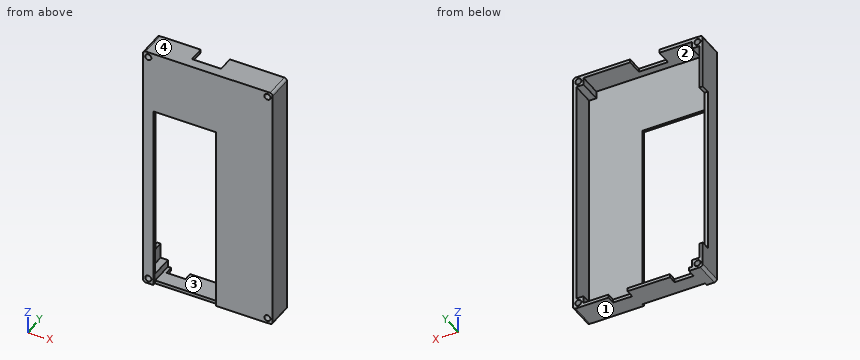
Autodesk Inventor part; units mm, degrees
ref_plane "YZ Plane" through (0, 0, 0) normal (1, 0, 0) x (0, 1, 0)
ref_plane "XZ Plane" through (0, 0, 0) normal (0, 1, 0) x (-1, 0, 0)
ref_plane "XY Plane" through (0, 0, 0) normal (0, 0, 1) x (1, 0, 0)
sketch "Sketch1" plane through (0, 0, 0) normal (0, 1, 0) x (-1, 0, 0)
  line L0 (0, 0) -> (62.23, 0)
  line L1 (62.23, 0) -> (62.23, -120.65)
  line L2 (62.23, -120.65) -> (0, -120.65)
  line L3 (0, -120.65) -> (0, 0)
  dimension "d0" = 62.23
  dimension "d1" = 120.65
extrude "Extrusion1" add sketch "Sketch1" along normal blind 1.5
sketch "Sketch2" plane through (0, 1.5, 0) normal (0, 1, 0) x (1, 0, 0)
  line L0 (-60.6425, 1.5875) -> (-1.5875, 1.5875)
  line L1 (-1.5875, 1.5875) -> (-1.5875, 119.0625)
  line L2 (-1.5875, 119.0625) -> (-60.6425, 119.0625)
  line L3 (-60.6425, 119.0625) -> (-60.6425, 1.5875)
  line L4 (-62.23, 0) -> (0, 0)
  line L5 (0, 0) -> (0, 120.65)
  line L6 (-62.23, 120.65) -> (-62.23, 0)
  line L7 (0, 120.65) -> (-62.23, 120.65)
  line L8 (0, 0) -> (-5.08, 0)
  line L9 (-5.08, 0) -> (-5.08, 5.08)
  line L10 (-5.08, 5.08) -> (0, 5.08)
  line L11 (0, 5.08) -> (0, 0)
  line L12 (-62.23, 0) -> (-57.15, 0)
  line L13 (-57.15, 0) -> (-57.15, 5.08)
  line L14 (-57.15, 5.08) -> (-62.23, 5.08)
  line L15 (-62.23, 5.08) -> (-62.23, 0)
  line L16 (0, 120.65) -> (-5.08, 120.65)
  line L17 (-5.08, 120.65) -> (-5.08, 115.57)
  line L18 (-5.08, 115.57) -> (0, 115.57)
  line L19 (0, 115.57) -> (0, 120.65)
  line L20 (-62.23, 120.65) -> (-57.15, 120.65)
  line L21 (-57.15, 120.65) -> (-57.15, 115.57)
  line L22 (-57.15, 115.57) -> (-62.23, 115.57)
  line L23 (-62.23, 115.57) -> (-62.23, 120.65)
  point P0 (0, 115.57)
  point P1 (-1.5875, 115.57)
  point P2 (-1.5875, 5.08)
  point P3 (-5.08, 1.5875)
  point P4 (-57.15, 1.5875)
  point P5 (-60.6425, 5.08)
  point P6 (-5.08, 119.0625)
  point P7 (-60.6425, 115.57)
  point P8 (-57.15, 119.0625)
  dimension "d4" = 1.5875
  dimension "d5" = 1.5875
  dimension "d6" = 1.5875
  dimension "d7" = 1.5875
  dimension "d8" = 5.08
  dimension "d9" = 5.08
  dimension "d10" = 5.08
  dimension "d11" = 5.08
  dimension "d12" = 5.08
  dimension "d13" = 5.08
  dimension "d14" = 5.08
  dimension "d15" = 5.08
extrude "Extrusion3" add sketch "Sketch2" along normal blind 9.525 contours L3 L14 L13 L0 | L0 L13 L4 L6 L14 L3 | L0 L9 L4 L13 | L14 L6 L22 L3 | L9 L10 L1 L0 | L0 L1 L10 L5 L4 L9 | L22 L6 L7 L21 L2 L3 | L3 L2 L21 L22 | L1 L18 L5 L10 | L21 L7 L17 L2 | L18 L17 L2 L1 | L1 L2 L17 L7 L5 L18
sketch "Sketch3" plane through (0, 11.025, 0) normal (0, 1, 0) x (1, 0, 0)
  line L0 (-62.23, 0) -> (0, 0)
  line L1 (-41.402, 0) -> (-27.432, 0)
  line L2 (-27.432, 0) -> (-27.432, 1.5875)
  line L3 (-27.432, 1.5875) -> (-41.402, 1.5875)
  line L4 (-41.402, 1.5875) -> (-41.402, 0)
  line L5 (0, 0) -> (0, 120.65)
  line L6 (-62.23, 120.65) -> (-62.23, 0)
  line L7 (0, 120.65) -> (-62.23, 120.65)
  line L8 (-60.6425, 115.57) -> (-60.6425, 5.08)
  line L9 (-62.23, 60.325) -> (-60.6425, 60.325)
  line L10 (-60.6425, 60.325) -> (-60.6425, 98.425)
  line L11 (-60.6425, 98.425) -> (-62.23, 98.425)
  line L12 (-62.23, 98.425) -> (-62.23, 60.325)
  point P0 (-59.69, 2.54)
  point P1 (-59.69, 118.11)
  point P2 (-2.54, 118.11)
  point P3 (-2.54, 2.54)
  dimension "d20" = 27.432
  dimension "d21" = 20.828
  dimension "d22" = 2.54
  dimension "d23" = 2.54
  dimension "d24" = 2.54
  dimension "d25" = 2.54
  dimension "d26" = 2.54
  dimension "d27" = 2.54
  dimension "d28" = 2.54
  dimension "d29" = 2.54
  dimension "d47" = 60.325
  dimension "d48" = 22.225
  dimension "d57" = 62.23
extrude "Extrusion4" cut sketch "Sketch3" against normal blind 7.5 contours L4 L3 L2 L0
sketch "Sketch5" plane through (0, 11.025, 0) normal (0, 1, 0) x (1, 0, 0)
  line L0 (-60.6425, 5.08) -> (-60.6425, 115.57)
  line L1 (-62.23, 120.65) -> (-62.23, 0)
  line L2 (-62.23, 108.204) -> (-60.6425, 108.204)
  line L3 (-62.23, 26.67) -> (-60.6425, 26.67)
  line L4 (-62.23, 0) -> (-41.402, 0)
  line L5 (0, 120.65) -> (-62.23, 120.65)
  point P0 (0, 0)
  dimension "d49" = 26.67
  dimension "d50" = 108.204
extrude "Extrusion5" cut sketch "Sketch5" against normal blind 4.35
sketch "Sketch6" plane through (0, 1.5, 0) normal (0, 1, 0) x (1, 0, 0)
  point P0 (0, 0)
extrude "Extrusion6" cut sketch "Sketch2" against normal through all contours L13 L14 L3 L22 L21 L2 L17 L18 L1 L10 L9 L0
sketch "Sketch7" plane through (0, 11.025, 0) normal (0, 1, 0) x (1, 0, 0)
  line L0 (-57.15, 119.0625) -> (-5.08, 119.0625)
  line L1 (-55.626, 119.0625) -> (-55.626, 120.65)
  line L2 (0, 120.65) -> (-62.23, 120.65)
  line L3 (-46.482, 119.0625) -> (-46.482, 120.65)
  line L4 (-62.23, 120.65) -> (-62.23, 108.204)
  line L5 (-26.162, 119.0625) -> (-26.162, 120.65)
  line L6 (-17.018, 119.0625) -> (-17.018, 120.65)
  point P0 (0, 0)
  dimension "d60" = 9.144
  dimension "d61" = 6.604
  dimension "d62" = 9.144
  dimension "d63" = 36.068
extrude "Extrusion7" cut sketch "Sketch7" against normal blind 4 contours L1 L2 L3 L0 | L5 L2 L6 L0
sketch "Sketch8" plane through (0, 0, 0) normal (0, -1, 0) x (1, 0, 0)
  line L0 (0, -120.65) -> (-62.23, -120.65)
  line L1 (-62.23, -120.65) -> (0, -120.65)
  line L2 (0, -120.65) -> (0, 0)
  line L3 (0, 0) -> (-62.23, 0)
  line L4 (-62.23, 0) -> (-62.23, -120.65)
extrude "Extrusion8" add sketch "Sketch8" along normal blind 1.27
sketch "Sketch9" plane through (0, -1.27, 0) normal (0, -1, 0) x (1, 0, 0)
  line L0 (-57.23, -120.65) -> (-27.23, -120.65)
  line L1 (-27.23, -120.65) -> (-27.23, -30)
  line L2 (-27.23, -30) -> (-57.23, -30)
  line L3 (-57.23, -30) -> (-57.23, -120.65)
  line L4 (0, 0) -> (-62.23, 0)
  line L5 (-62.23, 0) -> (-62.23, -120.65)
  dimension "d70" = 30
  dimension "d71" = 30
  dimension "d75" = 5
extrude "Extrusion9" cut sketch "Sketch9" against normal up to surface (1.27 mm away)
sketch "Sketch4" plane through (0, 11.025, 0) normal (0, 1, 0) x (1, 0, 0)
  line L0 (-27.432, 0) -> (0, 0)
  line L1 (0, 0) -> (0, 120.65)
  line L2 (-62.23, 0) -> (-41.402, 0)
  line L3 (-62.23, 120.65) -> (-62.23, 0)
  line L4 (0, 120.65) -> (-62.23, 120.65)
  point P0 (-2.54, 2.54)
  point P1 (-2.54, 118.11)
  point P2 (-59.69, 118.11)
  point P3 (-59.69, 2.54)
  dimension "d39" = 2.54
  dimension "d40" = 2.54
  dimension "d41" = 2.54
  dimension "d42" = 2.54
  dimension "d43" = 2.54
  dimension "d44" = 2.54
  dimension "d45" = 2.54
  dimension "d46" = 2.54
hole "Hole1" at (-2.54, 11.025, -2.54) at (-2.54, 11.025, -118.11) at (-59.69, 11.025, -118.11) at (-59.69, 11.025, -2.54) direction (0, -1, 0) diameter 2.9464 end through all
fillet "Fillet3" radius 1.27 4 edges at (0, 4.8775, -120.65) (0, 4.8775, 0) (-62.23, 4.8775, -120.65) (-62.23, 4.8775, 0)
equation "\"d4\" = d5"
equation "\"d6\" = d5"
equation "\"d7\" = d5"
equation "\"d10\" = d8"
equation "\"d11\" = d10"
equation "\"d12\" = d8"
equation "\"d13\" = d8"
equation "\"d14\" = d8"
equation "\"d15\" = d8"
equation "\"d62\" = d60"
properties part number "cover_top"
Design review of the part built by this model. Coordinates are the model's own, in mm. Face numbers are marked on the shaded views. A direction names the side the tool comes from. Coordinates: 2 decimals unless noted, no trailing zeros. Order: outer loops, then holes, each group sorted by start corner. A loop starts at its lowest first (then second) coordinate and runs counter-clockwise, first axis right, second up. Notation, with made-up numbers: (16, -17) - (71, -17) arc R21 ccw to (71, -9) - close; hole circle Ø2 at (2, 31). An arc over 180 degrees is marked (long way). One line per question, with ' | ' between items.
Q1. The part is to be moulded in two halves that separate along X. For the marked faces 1 and 2, say which applies: +X half, -X half, draft (parallel to the pull), parting line (faces both ways), or undercut.
Answer key:
face 1: draft | face 2: undercut
Q2. Consider section C-C, the plane z = -63. Give the boundary of the cut face in (x, y) (1 decimal), then the cut area to 3 significant figures.
Answer key:
outline: (-62.2, -1.3) - (-57.2, -1.3) - (-57.2, 0) - (-60.6, 0) - (-60.6, 6.7) - (-62.2, 6.7) - close; (-27.2, -1.3) - (0, -1.3) - (0, 11) - (-1.6, 11) - (-1.6, 0) - (-27.2, 0) - close | area: 69.0 mm2
Q3. Consider section D-D, the plane z = -10. Give the boundary of the cut face in (x, y) (1 decimal), then the cut area to 3 significant figures.
Answer key:
outline: (-62.2, -1.3) - (0, -1.3) - (0, 11) - (-1.6, 11) - (-1.6, 0) - (-60.6, 0) - (-60.6, 11) - (-62.2, 11) - close | area: 114 mm2
Q4. Consider section A-A, the plane y = 2.25. Give the boundary of the cut face in (x, z), then the cut area to 3 significant figures.
Answer key:
outline: (-62.23, -119.38) arc R1.27 ccw to (-60.96, -120.65) - (-1.27, -120.65) arc R1.27 ccw to (0, -119.38) - (0, -1.27) arc R1.27 ccw to (-1.27, 0) - (-60.96, 0) arc R1.27 ccw to (-62.23, -1.27) - close; hole circle Ø2.95 at (-59.69, -118.11); hole circle Ø2.95 at (-59.69, -2.54); hole (-60.64, -115.57) - (-57.15, -115.57) - (-57.15, -119.06) - (-5.08, -119.06) - (-5.08, -115.57) - (-1.59, -115.57) - (-1.59, -5.08) - (-5.08, -5.08) - (-5.08, -1.59) - (-57.15, -1.59) - (-57.15, -5.08) - (-60.64, -5.08) - close; hole circle Ø2.95 at (-2.54, -118.11); hole circle Ø2.95 at (-2.54, -2.54) | area: 591 mm2
Q5. For the marked faces 3 and 4, list the 3-axis set-ups (+Z, -Z, +X, -X, +Y, -Y) from which the entire face can be reached by the end or side of a thin tool; tool diameter is ignored.
Answer key:
face 3: +Y | face 4: +Z, +X, -X, +Y, -Y
Q6. Clearance check with flat-ended pins moving along their axes: pin 1 Ø5.5 at (x, z) = (-46.5, -118.5) entering from -Y; pin 2 Ø1.3 at (x, z) = (-62, -63.5) entering from +Y (3 decimals); pin 3 Ø0.5 at (y, z) = (9, -0.5) entering from +X. State where each tip first meets the part, or that it passes through.
Answer key:
pin 1: stops at y = 0 | pin 2: stops at y = 6.675 | pin 3: stops at x = -0.11
Q7. To check wall thickness, follow line 1 along Z through (x, y) = (-2.54, 8.25); line 2 along X through (y, z) = (3.25, -2.54); line 3 along X through (y, z) = (4.5, -34). State the ranges of each line that lie inside material, in increasing order.
Answer key:
line 1: z = -120.65 to -119.58, -116.64 to -115.57, -5.08 to -4.01, -1.07 to 0 | line 2: x = -62.23 to -61.16, -58.22 to -57.15, -5.08 to -4.01, -1.07 to 0 | line 3: x = -62.23 to -60.64, -1.59 to 0
